CAD build for the part. Positions are in the model's coordinates, mm. A direction names the side the tool comes from. Coordinates: 2 decimals unless noted, no trailing zeros. Order: outer loops, then holes, each group sorted by start corner. A loop starts at its lowest first (then second) coordinate and runs counter-clockwise, first axis right, second up. Notation, with made-up numbers: (24, 83.5) - (68, 83.5) arc R29 ccw to (68, 118.5) - close; hole circle Ø8 at (51, -19.5). An arc over 180 degrees is marked (long way). Return JSON: item names as keys, results as strings.
from build123d import *

# Parameters (mm, degrees)
F0_W           = 90
F0_H           = 159
F1_DEPTH       = 7.5
F3_D           = 6.6
F3_CBORE_D     = 11.25
F3_CBORE_DEPTH = 6
F5_D           = 6.6
F5_CBORE_D     = 11.25
F5_CBORE_DEPTH = 6
F7_D           = 9
F7_DEPTH       = 2
F7_TIP         = 2.7038727856


with BuildPart() as f1:
    # F0 (on Front) → F1 (new body, symmetric)
    with BuildSketch(Plane.XZ):
        Rectangle(F0_W, F0_H)
    extrude(amount=F1_DEPTH, both=True)

    # F3 (through all)
    with Locations(Plane.XZ.offset(7.5)):
        with Locations((-25, 69.5), (25, 69.5), (-25, -69.5), (25, -69.5)):
            CounterBoreHole(F3_D / 2, F3_CBORE_D / 2, F3_CBORE_DEPTH)

    # F5 (through all)
    with Locations(Plane(origin=(0, 7.5, 0), x_dir=(-1, 0, 0), z_dir=(0, 1, 0))):
        with Locations((-15, 45), (15, 45), (15, -45), (-15, -45)):
            CounterBoreHole(F5_D / 2, F5_CBORE_D / 2, F5_CBORE_DEPTH)

    # F7
    with Locations(Plane.XZ.offset(7.5)):
        with Locations((-15, 45), (15, 45), (-15, -45), (15, -45)):
            Hole(F7_D / 2, depth=F7_DEPTH)
            with Locations((0, 0, -(F7_DEPTH + F7_TIP / 2))):  # 118° drill point
                Cone(0, F7_D / 2, F7_TIP, mode=Mode.SUBTRACT)


solid = f1.part
Item 1: Band-saw the part on A-A, the plane x = -15. List the corners of the cut face in (y, z) (3 decimals).
Findings below:
{"outline": "(-7.5, -79.5) - (7.5, -79.5) - (7.5, -50.625) - (1.5, -50.625) - (1.5, -48.3) - (-4.779, -48.3) - (-5.5, -49.5) - (-7.5, -49.5) - close; (-7.5, -40.5) - (-5.5, -40.5) - (-4.779, -41.7) - (1.5, -41.7) - (1.5, -39.375) - (7.5, -39.375) - (7.5, 39.375) - (1.5, 39.375) - (1.5, 41.7) - (-4.779, 41.7) - (-5.5, 40.5) - (-7.5, 40.5) - close; (-7.5, 49.5) - (-5.5, 49.5) - (-4.779, 48.3) - (1.5, 48.3) - (1.5, 50.625) - (7.5, 50.625) - (7.5, 79.5) - (-7.5, 79.5) - close"}
Item 2: Which spindle directions (+Z, -Z, +X, -X, +Y, -Y) get a long thin tool onto all of the face, cutting with end or side? Do faces 1 (the cylindrical face through (-26.774, 3.063, -66.717)), 2 (the cylindrical face through (15.732, 4.542, 50.577)), 3 (the cylindrical face through (-29.15, -4.54, -65.7)). Say none if no direction does.
Findings below:
{"face 1": "+Y, -Y", "face 2": "+Y", "face 3": "-Y"}
Item 3: Band-saw the part on C-C, the plane z = 45. List the corners of the cut face in (x, y) (3 decimals), then the cut area to 3 significant figures.
Findings below:
{"outline": "(-45, -7.5) - (-19.5, -7.5) - (-19.5, -5.5) - (-18.3, -4.779) - (-18.3, 1.5) - (-20.625, 1.5) - (-20.625, 7.5) - (-45, 7.5) - close; (-11.7, -4.779) - (-10.5, -5.5) - (-10.5, -7.5) - (10.5, -7.5) - (10.5, -5.5) - (11.7, -4.779) - (11.7, 1.5) - (9.375, 1.5) - (9.375, 7.5) - (-9.375, 7.5) - (-9.375, 1.5) - (-11.7, 1.5) - close; (18.3, -4.779) - (19.5, -5.5) - (19.5, -7.5) - (45, -7.5) - (45, 7.5) - (20.625, 7.5) - (20.625, 1.5) - (18.3, 1.5) - close", "area": "1,080 mm²"}
Item 4: Wall check: L1, parallel to Z at x = 25, y = -5.3 (3 decimals); L2, parallel to Z at x = -25, y = 1.5; L3, parallel to X at y = 2.75, z = -46. Give the ranges that are in metal, low to high. Write a range as [from, to].
Findings below:
{"L1": "z = [-79.5, -75.125], [-63.875, 63.875], [75.125, 79.5]", "L2": "z = [-79.5, -72.8], [-66.2, 66.2], [72.8, 79.5]", "L3": "x = [-45, -20.54], [-9.46, 9.46], [20.54, 45]"}
Item 5: Mould opens along X. For faces 4 (the cylindrical face through (-26.774, 3.063, 72.283)), 5 (the flat face through (-1, -7.5, 1)) say: released by +X, released by -X, zero draft, split by the parting line, or undercut.
Findings below:
{"face 4": "undercut", "face 5": "zero draft"}
Item 6: Band-saw the part on B-B, the plane z = -69.5. List the corners of the cut face in (x, y) (3 decimals).
Findings below:
{"outline": "(-45, -7.5) - (-30.625, -7.5) - (-30.625, -1.5) - (-28.3, -1.5) - (-28.3, 7.5) - (-45, 7.5) - close; (-21.7, -1.5) - (-19.375, -1.5) - (-19.375, -7.5) - (19.375, -7.5) - (19.375, -1.5) - (21.7, -1.5) - (21.7, 7.5) - (-21.7, 7.5) - close; (28.3, -1.5) - (30.625, -1.5) - (30.625, -7.5) - (45, -7.5) - (45, 7.5) - (28.3, 7.5) - close"}
Item 7: Drop flat-ended pins along their axis: P1, Ø10.5, axis at x = 15, z = -45, coming from the -Y side; P2, Ø3.5, axis at x = -26.5, z = -67.5, coming from the -Y side; P3, Ø8.5, axis at x = -15, z = -45, coming from the +Y side; P4, Ø8, axis at x = 15, z = -45, coming from the -Y side. Give the stop position or say it passes through.
Findings below:
{"P1": "stops at y = -7.5", "P2": "stops at y = -1.5", "P3": "stops at y = 1.5", "P4": "stops at y = -5.2"}
